Check sheet for the modelled part. Datum: model origin and axes. Units: mm. A direction names the side the tool comes from. Round coordinates to 2 decimals unless told otherwise and drop trailing zeros. Loops run counter-clockwise (first coordinate to the right, second up) from the corner with the lowest first, then second, coordinate; pieces in that order, holes last. Notation, with made-up numbers: (-22, 36) -> (32, 36) arc R27 cw to (32, 52) -> close; hole circle Ø10 at (16.25, 36.5). An arc over 180 degrees is marked (long way). Use one line per item in the form item = value. Start each with the question number.
(1) Set-up check for faces 5 (the flat face through (-27, 12.224, 20)), 6 (the flat face through (23.726, -3.32, 6.409)), 7 (the flat face through (-23.726, 15.467, 22.888)): record each of +Z, -Z, +X, -X, +Y, -Y from which the full face is reachable in a straight line by a thin tool's end or side.
(2) Sectioned sample at A-A (z = 7). Record the cut outline in (x, y).
(3) Draft check along X on faces 1 (the cylindrical face through (-0.316, -8.046, 6.409)), 2 (the flat face through (-27, -0.077, 20)), 3 (the flat face through (26.245, 17.191, 14.79)), 4 (the flat face through (-23.726, 15.467, 6.409)). Enter one of: released by +X, released by -X, zero draft, split by the parting line, or undercut.
(4) Sectioned sample at B-B (y = 9). Record the cut outline in (x, z), and give its area (3 significant figures).
(5) Sectioned sample at C-C (z = 26). Record the cut outline in (x, y), and give its area (3 significant figures).
(6) Material ranges on probe 1 along Z at (x, y) = (21, 14); probe 2 along X at (y, z) = (0, 16.5); probe 3 along X at (y, z) = (5, 24.5), recorded low to high. Write a range as [from, to].
(7) Go/stop test with flat-tipped pins: pin 1 (1.3 mm diameter, centred on x = 6, y = 6.5, fed in from -Z); pin 2 (1.5 mm diameter, centred on y = 23, z = 13, fed in from -X); pin 3 (2 mm diameter, centred on x = -6, z = 22, fed in from +Y). Record where each tip stops, or that it passes through.
from build123d import *

# Parameters (mm, degrees)
F0_R      = 4.5
F0_R_2    = 2.15
F1_DEPTH  = 33
F2_DEPTH  = 31
F3_DEPTH  = 15
F4_DEPTH  = 13
F5_DEPTH  = 31
F6_R      = 3
F7_DEPTH  = 24
F8_W      = 6.3
F8_H      = 5
F9_DEPTH  = 4
F10_W     = 12.3
F10_H     = 5
F11_DEPTH = 4


with BuildPart() as f1:
    # F0 (on Top) → F1 (new body)
    with BuildSketch(Plane.XY):
        with BuildLine():
            Line((28.25, -3.038874), (28.25, 15.186))
            Line((28.25, 15.186), (24.182373, 19.253627))
            ThreePointArc((24.182373, 19.253627), (0, 26.943359), (-24.182373, 19.253627))
            Line((-24.182373, 19.253627), (-28.25, 15.186))
            Line((-28.25, 15.186), (-28.25, -3.038874))
            Line((-28.25, -3.038874), (-23.834695, -7.454179))
            ThreePointArc((-23.834695, -7.454179), (0, -11.046233), (23.834695, -7.454179))
            Line((23.834695, -7.454179), (28.25, -3.038874))
        make_face()
        with BuildLine():
            Line((-22.244796, -4.801437), (-25.25, -1.796233))
            Line((-25.25, -1.796233), (-25.25, 13.943359))
            Line((-25.25, 13.943359), (-22.244796, 16.948563))
            ThreePointArc((-22.244796, 16.948563), (0, 23.943359), (22.244796, 16.948563))
            Line((22.244796, 16.948563), (25.25, 13.943359))
            Line((25.25, 13.943359), (25.25, -1.796233))
            Line((25.25, -1.796233), (22.244796, -4.801437))
            ThreePointArc((22.244796, -4.801437), (0, -8.046233), (-22.244796, -4.801437))
        make_face(mode=Mode.SUBTRACT)
        with BuildLine():
            Line((-25.25, 13.943359), (-25.25, -1.796233))
            Line((-25.25, -1.796233), (-22.244796, -4.801437))
            ThreePointArc((-22.244796, -4.801437), (0, -8.046233), (22.244796, -4.801437))
            Line((22.244796, -4.801437), (25.25, -1.796233))
            Line((25.25, -1.796233), (25.25, 13.943359))
            Line((25.25, 13.943359), (22.244796, 16.948563))
            ThreePointArc((22.244796, 16.948563), (0, 23.943359), (-22.244796, 16.948563))
            Line((-22.244796, 16.948563), (-25.25, 13.943359))
        make_face()
        with BuildLine():
            Line((20.314515, 14.636203), (22.25, 12.700719))
            Line((22.25, 12.700719), (22.25, -1.663785))
            ThreePointArc((22.25, -1.663785), (0, -5.046233), (-22.25, -1.663785))
            Line((-22.25, -1.663785), (-22.25, 12.700719))
            Line((-22.25, 12.700719), (-20.314515, 14.636203))
            ThreePointArc((-20.314515, 14.636203), (0, 20.943359), (20.314515, 14.636203))
        make_face(mode=Mode.SUBTRACT)
        with BuildLine():
            Line((22.25, -1.663785), (22.25, 12.700719))
            Line((22.25, 12.700719), (20.314515, 14.636203))
            ThreePointArc((20.314515, 14.636203), (0, 20.943359), (-20.314515, 14.636203))
            Line((-20.314515, 14.636203), (-22.25, 12.700719))
            Line((-22.25, 12.700719), (-22.25, -1.663785))
            ThreePointArc((-22.25, -1.663785), (0, -5.046233), (22.25, -1.663785))
        make_face()
        with Locations((6.75, 6.073359)):
            Circle(F0_R, mode=Mode.SUBTRACT)
        with Locations((6.75, 6.073359)):
            Circle(F0_R)
        with Locations((6.75, 6.073359)):
            Circle(F0_R_2, mode=Mode.SUBTRACT)
        with Locations((6.75, 6.073359)):
            Circle(F0_R_2)
    extrude(amount=F1_DEPTH)

    # F0 (on Top) → F2 (cut)
    with BuildSketch(Plane.XY):
        with BuildLine():
            Line((-25.25, 13.943359), (-25.25, -1.796233))
            Line((-25.25, -1.796233), (-22.244796, -4.801437))
            ThreePointArc((-22.244796, -4.801437), (0, -8.046233), (22.244796, -4.801437))
            Line((22.244796, -4.801437), (25.25, -1.796233))
            Line((25.25, -1.796233), (25.25, 13.943359))
            Line((25.25, 13.943359), (22.244796, 16.948563))
            ThreePointArc((22.244796, 16.948563), (0, 23.943359), (-22.244796, 16.948563))
            Line((-22.244796, 16.948563), (-25.25, 13.943359))
        make_face()
        with BuildLine():
            Line((20.314515, 14.636203), (22.25, 12.700719))
            Line((22.25, 12.700719), (22.25, -1.663785))
            ThreePointArc((22.25, -1.663785), (0, -5.046233), (-22.25, -1.663785))
            Line((-22.25, -1.663785), (-22.25, 12.700719))
            Line((-22.25, 12.700719), (-20.314515, 14.636203))
            ThreePointArc((-20.314515, 14.636203), (0, 20.943359), (20.314515, 14.636203))
        make_face(mode=Mode.SUBTRACT)
        with BuildLine():
            Line((22.25, -1.663785), (22.25, 12.700719))
            Line((22.25, 12.700719), (20.314515, 14.636203))
            ThreePointArc((20.314515, 14.636203), (0, 20.943359), (-20.314515, 14.636203))
            Line((-20.314515, 14.636203), (-22.25, 12.700719))
            Line((-22.25, 12.700719), (-22.25, -1.663785))
            ThreePointArc((-22.25, -1.663785), (0, -5.046233), (22.25, -1.663785))
        make_face()
        with Locations((6.75, 6.073359)):
            Circle(F0_R, mode=Mode.SUBTRACT)
    extrude(amount=F2_DEPTH, mode=Mode.SUBTRACT)

    # F0 (on Top) → F3 (join)
    with BuildSketch(Plane.XY):
        with BuildLine():
            Line((-25.25, 13.943359), (-25.25, -1.796233))
            Line((-25.25, -1.796233), (-22.244796, -4.801437))
            ThreePointArc((-22.244796, -4.801437), (0, -8.046233), (22.244796, -4.801437))
            Line((22.244796, -4.801437), (25.25, -1.796233))
            Line((25.25, -1.796233), (25.25, 13.943359))
            Line((25.25, 13.943359), (22.244796, 16.948563))
            ThreePointArc((22.244796, 16.948563), (0, 23.943359), (-22.244796, 16.948563))
            Line((-22.244796, 16.948563), (-25.25, 13.943359))
        make_face()
        with BuildLine():
            Line((20.314515, 14.636203), (22.25, 12.700719))
            Line((22.25, 12.700719), (22.25, -1.663785))
            ThreePointArc((22.25, -1.663785), (0, -5.046233), (-22.25, -1.663785))
            Line((-22.25, -1.663785), (-22.25, 12.700719))
            Line((-22.25, 12.700719), (-20.314515, 14.636203))
            ThreePointArc((-20.314515, 14.636203), (0, 20.943359), (20.314515, 14.636203))
        make_face(mode=Mode.SUBTRACT)
    extrude(amount=F3_DEPTH)

    # F0 (on Top) → F4 (cut)
    with BuildSketch(Plane.XY):
        with BuildLine():
            Line((-25.25, 13.943359), (-25.25, -1.796233))
            Line((-25.25, -1.796233), (-22.244796, -4.801437))
            ThreePointArc((-22.244796, -4.801437), (0, -8.046233), (22.244796, -4.801437))
            Line((22.244796, -4.801437), (25.25, -1.796233))
            Line((25.25, -1.796233), (25.25, 13.943359))
            Line((25.25, 13.943359), (22.244796, 16.948563))
            ThreePointArc((22.244796, 16.948563), (0, 23.943359), (-22.244796, 16.948563))
            Line((-22.244796, 16.948563), (-25.25, 13.943359))
        make_face()
        with BuildLine():
            Line((20.314515, 14.636203), (22.25, 12.700719))
            Line((22.25, 12.700719), (22.25, -1.663785))
            ThreePointArc((22.25, -1.663785), (0, -5.046233), (-22.25, -1.663785))
            Line((-22.25, -1.663785), (-22.25, 12.700719))
            Line((-22.25, 12.700719), (-20.314515, 14.636203))
            ThreePointArc((-20.314515, 14.636203), (0, 20.943359), (20.314515, 14.636203))
        make_face(mode=Mode.SUBTRACT)
    extrude(amount=F4_DEPTH, mode=Mode.SUBTRACT)

    # F0 (on Top) → F5 (cut)
    with BuildSketch(Plane.XY):
        with Locations((6.75, 6.073359)):
            Circle(F0_R_2)
    extrude(amount=F5_DEPTH, mode=Mode.SUBTRACT)

    # F6
    f6_edges = [f1.edges().sort_by_distance(p)[0] for p in [
        (0, -11.046233, 33),
        (-28.25, 6.073563, 33),
        (0, 26.943359, 33),
        (28.25, 6.073563, 33),
        (-26.042347, -5.246526, 33),
        (26.042347, -5.246526, 33),
        (26.216187, 17.219813, 33),
        (-26.216187, 17.219813, 33),
    ]]
    fillet(f6_edges, radius=F6_R)

    # F0 (on Top) → F7 (cut)
    with BuildSketch(Plane.XY):
        with Locations((6.75, 6.073359)):
            Circle(F0_R)
        with Locations((6.75, 6.073359)):
            Circle(F0_R_2, mode=Mode.SUBTRACT)
        with Locations((6.75, 6.073359)):
            Circle(F0_R_2)
    extrude(amount=F7_DEPTH, mode=Mode.SUBTRACT)

    # F8 (on face) → F9 (cut)
    with BuildSketch(Plane.YZ.offset(28.25)):
        with Locations((4.111126, 27.5)):
            Rectangle(F8_W, F8_H)
    extrude(amount=-F9_DEPTH, mode=Mode.SUBTRACT)

    # F10 (on face) → F11 (cut)
    with BuildSketch(Plane(origin=(-28.25, 0, 0), x_dir=(0, -1, 0), z_dir=(-1, 0, 0))):
        with Locations((-6.0735, 20.5)):
            Rectangle(F10_W, F10_H)
    extrude(amount=-F11_DEPTH, mode=Mode.SUBTRACT)


solid = f1.part
Checks:
q1.face_5 = -X
q1.face_6 = -Z
q1.face_7 = none
q2.outline = (-28.25, -3.04) -> (-23.83, -7.45) arc R80.87 ccw to (23.83, -7.45) -> (28.25, -3.04) -> (28.25, 15.19) -> (24.18, 19.25) arc R41.87 ccw to (-24.18, 19.25) -> (-28.25, 15.19) -> close; hole (-25.25, -1.8) -> (-22.24, -4.8) arc R77.87 ccw to (22.24, -4.8) -> (25.25, -1.8) -> (25.25, 13.94) -> (22.24, 16.95) arc R38.87 ccw to (-22.24, 16.95) -> (-25.25, 13.94) -> close
q3.face_1 = undercut
q3.face_2 = zero draft
q3.face_3 = released by +X
q3.face_4 = undercut
q4.outline = (-28.25, 0) -> (-25.25, 0) -> (-25.25, 13) -> (-22.25, 13) -> (-22.25, 15) -> (-25.25, 15) -> (-25.25, 18) -> (-28.25, 18) -> close; (-28.25, 23) -> (-25.25, 23) -> (-25.25, 31) -> (3.33, 31) -> (3.33, 24) -> (10.17, 24) -> (10.17, 31) -> (25.25, 31) -> (25.25, 15) -> (22.25, 15) -> (22.25, 13) -> (25.25, 13) -> (25.25, 0) -> (28.25, 0) -> (28.25, 30) arc R3 ccw to (25.25, 33) -> (-25.25, 33) arc R3 ccw to (-28.25, 30) -> close
q4.area = 340 mm2
q5.outline = (-28.25, -3.04) -> (-23.83, -7.45) arc R80.87 ccw to (23.83, -7.45) -> (28.25, -3.04) -> (28.25, 0.96) -> (25.25, 0.96) -> (25.25, -1.8) -> (22.24, -4.8) arc R77.87 cw to (-22.24, -4.8) -> (-25.25, -1.8) -> (-25.25, 13.94) -> (-22.24, 16.95) arc R38.87 cw to (22.24, 16.95) -> (25.25, 13.94) -> (25.25, 7.26) -> (28.25, 7.26) -> (28.25, 15.19) -> (24.18, 19.25) arc R41.87 ccw to (-24.18, 19.25) -> (-28.25, 15.19) -> close; circle Ø9 at (6.75, 6.07); hole circle Ø4.3 at (6.75, 6.07)
q5.area = 482 mm2
q6.probe_1 = [13, 15], [31, 33]
q6.probe_2 = [-28.25, -25.25], [25.25, 28.25]
q6.probe_3 = [-28.25, -25.25], [2.38, 4.89], [8.61, 11.12], [25.25, 28.25]
q7.pin_1 = 31
q7.pin_2 = -19.26
q7.pin_3 = 26.64
